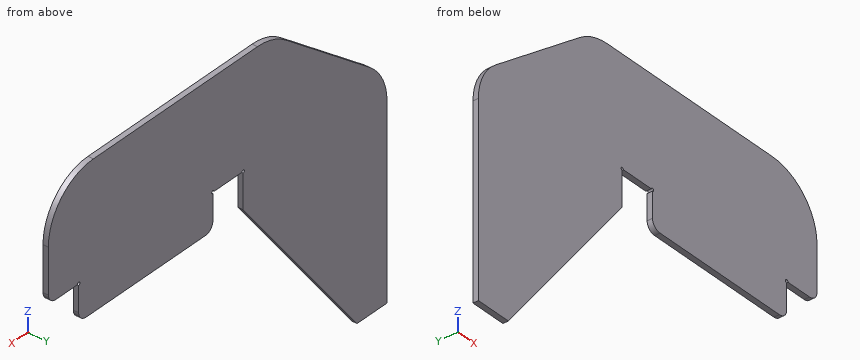
from build123d import *

# Parameters (mm, degrees)
SKETCH1_W           = 150
SKETCH1_H           = 60
BOSS_EXTRUDE1_DEPTH = 3
FILLET1_R           = 30
SKETCH2_W           = 89.6
SKETCH2_H           = 20
BOSS_EXTRUDE2_DEPTH = 3
FILLET2_R           = 30
SKETCH3_R           = 0.8
SKETCH3_R_2         = 0.899402105
CUT_EXTRUDE1_DEPTH  = 160.091168831
FILLET3_R           = 5
SKETCH4_W           = 20
SKETCH4_H           = 100
BOSS_EXTRUDE3_DEPTH = 3
BOSS_EXTRUDE4_DEPTH = 3


with BuildPart() as part:
    # Sketch1 → Boss-Extrude1 (new body)
    with BuildSketch(Plane(origin=(0, 0, 0), x_dir=(1, 0, 0), z_dir=(0, 1, 0))):
        Rectangle(SKETCH1_W, SKETCH1_H)
    extrude(amount=BOSS_EXTRUDE1_DEPTH)

    # Fillet1
    fillet1_edges = [part.edges().sort_by_distance(p)[0] for p in [
        (75, 1.5, 30),
    ]]
    fillet(fillet1_edges, radius=FILLET1_R)

    # Sketch2 → Boss-Extrude2 (add)
    with BuildSketch(Plane(origin=(0, 3, 0), x_dir=(1, 0, 0), z_dir=(0, 1, 0))):
        Polygon((-75, 30), (-55, 30), (-55, 50), (-151, 50), (-151, 30), align=None)
        Polygon((-75, -30), (-75, 30), (-151, 30), align=None)
        with Locations((10, 40)):
            Rectangle(SKETCH2_W, SKETCH2_H)
    extrude(amount=-BOSS_EXTRUDE2_DEPTH)

    # Fillet2
    fillet2_edges = [part.edges().sort_by_distance(p)[0] for p in [
        (-151, 1.5, -30),
        (-75, 1.5, 30),
    ]]
    fillet(fillet2_edges, radius=FILLET2_R)

    # Sketch3 → Cut-Extrude1 (cut, through all)
    with BuildSketch(Plane(origin=(0, 3, 0), x_dir=(1, 0, 0), z_dir=(0, 1, 0))):
        with Locations((-55, 30)):
            Circle(SKETCH3_R)
        with Locations((-34.8, 30)):
            Circle(SKETCH3_R)
        with Locations((54.8, 30)):
            Circle(SKETCH3_R_2)
    extrude(amount=-CUT_EXTRUDE1_DEPTH, mode=Mode.SUBTRACT)

    # Fillet3
    fillet3_edges = [part.edges().sort_by_distance(p)[0] for p in [
        (-34.8, 1.5, -50),
        (54.8, 1.5, -50),
        (75, 1.5, -30),
    ]]
    fillet(fillet3_edges, radius=FILLET3_R)

    # Sketch4 → Boss-Extrude3 (add)
    with BuildSketch(Plane(origin=(0, 0, 0), x_dir=(-1, 0, 0), z_dir=(0, -1, 0))):
        with Locations((141, 100)):
            Rectangle(SKETCH4_W, SKETCH4_H)
    extrude(amount=-BOSS_EXTRUDE3_DEPTH)

    # Sketch5 → Boss-Extrude4 (add)
    with BuildSketch(Plane(origin=(0, 3, 0), x_dir=(1, 0, 0), z_dir=(0, 1, 0))):
        Polygon((-131, 150), (-55, 50), (-131, 50), align=None)
    extrude(amount=-BOSS_EXTRUDE4_DEPTH)


solid = part.part
The listing builds one solid part. Answer for the finished solid, in the listing's coordinates (mm). Give positions to 0.01 mm unless a question says otherwise; leave off trailing zeros. Write each loop counter-clockwise with the first axis right and the second up, starting at its lowest first coordinate (ties: lowest second). Pieces come first, ordered by that corner, then holes.
Item 1: Flat-ended cylindrical pins translate along their axes: P1, Ø2, axis at x = 54.8, z = -30, coming from the +Y side; P2, Ø1.3, axis at x = -34.8, z = -30, coming from the +Y side; P3, Ø0.9, axis at y = 2, z = -39, coming from the +X side; P4, Ø1, axis at y = 2, z = -12.5, coming from the -X side. Find the tip coordinate at first contact, or state that the pin passes through.
Item 2: Find the intervals of material crossed by line 1 along Z through (x, y) = (-1, 0.7); line 2 along Z through (x, y) = (-45, 0.4); line 3 along X through (y, z) = (2.75, -7), in increasing order.
Item 3: Section A-A, the plane y = 1.15 is taken. Write down the section's boundary in (x, z), plus the area to 3 significant figures.
Item 4: Section C-C, the plane x = -23 is taken. Write down the section's boundary in (y, z).
Item 5: Section B-B, the plane z = -129 is taken. Write down the section's boundary in (x, y), plus the area to 3 significant figures.
Completed:
1. P1: stops at y = 3
1. P2: passes through
1. P3: stops at x = 54.8
1. P4: stops at x = -129.47
2. line 1: z = -50 to 30
2. line 2: z = -30 to 30
2. line 3: x = -121.87 to 75
3. outline: (-151, -150) - (-131, -150) - (-55, -50) - (-55, -30.8) arc R0.8 cw (long way) to (-54.2, -30) - (-35.6, -30) arc R0.8 cw (long way) to (-34.8, -30.8) - (-34.8, -45) arc R5 ccw to (-29.8, -50) - (49.8, -50) arc R5 ccw to (54.8, -45) - (54.8, -30.9) arc R0.9 cw (long way) to (55.7, -30) - (70, -30) arc R5 ccw to (75, -25) - (75, 0) arc R30 ccw to (45, 30) - (-64.59, 30) arc R30 ccw to (-83.17, 23.55) - (-139.59, -20.99) arc R30 ccw to (-151, -44.54) - close
3. area: 20,500 mm2
4. outline: (0, -50) - (3, -50) - (3, 30) - (0, 30) - close
5. outline: (-151, 0) - (-115.04, 0) - (-115.04, 3) - (-151, 3) - close
5. area: 108 mm2
